```python
from build123d import *

# Parameters (mm, degrees)
ESBO_O2_R                = 8.85
RESSALTO_EXTRUS_O1_DEPTH = 6.4
ESBO_O3_R                = 8.25
CORTE_EXTRUS_O1_DEPTH    = 5
ESBO_O4_R                = 7.75
RESSALTO_EXTRUS_O2_DEPTH = 9
FILETE1_R                = 0.2
ESBO_O5_R                = 7.8
RESSALTO_EXTRUS_O3_DEPTH = 11
ESBO_O6_R                = 7.25
RESSALTO_EXTRUS_O4_DEPTH = 10.3
ESBO_O7_W                = 21.473826642
ESBO_O7_H                = 23.10287556
CORTE_EXTRUS_O2_DEPTH    = 11
ESBO_O8_W                = 2.8
ESBO_O8_H                = 0.5
RESSALTO_EXTRUS_O5_DEPTH = 8


with BuildPart() as part:
    # Esboço2 → Ressalto-extrusão1 (new body)
    with BuildSketch(Plane(origin=(0, 0, 0), x_dir=(1, 0, 0), z_dir=(0, 1, 0))):
        Circle(ESBO_O2_R)
    extrude(amount=RESSALTO_EXTRUS_O1_DEPTH)

    # Esboço3 → Corte-extrusão1 (cut)
    with BuildSketch(Plane(origin=(0, 6.4, 0), x_dir=(1, 0, 0), z_dir=(0, 1, 0))):
        Circle(ESBO_O3_R)
    extrude(amount=-CORTE_EXTRUS_O1_DEPTH, mode=Mode.SUBTRACT)

    # Esboço4 → Ressalto-extrusão2 (add)
    with BuildSketch(Plane(origin=(0, 1.4, 0), x_dir=(1, 0, 0), z_dir=(0, 1, 0))):
        Circle(ESBO_O4_R)
    extrude(amount=RESSALTO_EXTRUS_O2_DEPTH)

    # Filete1
    filete1_edges = [part.edges().sort_by_distance(p)[0] for p in [
        (-7.75, 10.4, 0),
        (-8.85, 6.4, 0),
    ]]
    fillet(filete1_edges, radius=FILETE1_R)

    # Esboço5 → Ressalto-extrusão3 (add)
    with BuildSketch(Plane.XZ):
        Circle(ESBO_O5_R)
    extrude(amount=RESSALTO_EXTRUS_O3_DEPTH)

    # Esboço6 → Ressalto-extrusão4 (add)
    with BuildSketch(Plane.XZ.offset(11)):
        Circle(ESBO_O6_R)
    extrude(amount=RESSALTO_EXTRUS_O4_DEPTH)

    # Esboço7 → Corte-extrusão2 (cut)
    with BuildSketch(Plane.XZ.offset(11)):
        Rectangle(ESBO_O7_W, ESBO_O7_H)
        Polygon((-7.25, -7.8), (-1, -7.8), (-1, -7.25), (1, -7.25), (1, -7.8), (7.25, -7.8), (7.25, 7.8), (1, 7.8), (1, 7.25), (-1, 7.25), (-1, 7.8), (-7.25, 7.8), align=None, mode=Mode.SUBTRACT)
    extrude(amount=-CORTE_EXTRUS_O2_DEPTH, mode=Mode.SUBTRACT)

    # Esboço8 → Ressalto-extrusão5 (add)
    with BuildSketch(Plane.XZ.offset(21.3)):
        with Locations((-5, 2.75)):
            Rectangle(ESBO_O8_W, ESBO_O8_H)
        with Locations((0, 2.75)):
            Rectangle(ESBO_O8_W, ESBO_O8_H)
        with Locations((5, 2.75)):
            Rectangle(ESBO_O8_W, ESBO_O8_H)
        with Locations((0, 6.25)):
            Rectangle(ESBO_O8_W, ESBO_O8_H)
        with Locations((0, -6.25)):
            Rectangle(ESBO_O8_W, ESBO_O8_H)
        with Locations((5, -2.75)):
            Rectangle(ESBO_O8_W, ESBO_O8_H)
        with Locations((0, -2.75)):
            Rectangle(ESBO_O8_W, ESBO_O8_H)
        with Locations((-5, -2.75)):
            Rectangle(ESBO_O8_W, ESBO_O8_H)
    extrude(amount=RESSALTO_EXTRUS_O5_DEPTH)


solid = part.part
```
The model under review builds one solid part; all positions refer to its coordinate system, in mm. A direction names the side the tool comes from. Round coordinates to 2 decimals unless told otherwise and drop trailing zeros. Order: outer loops, then holes, each group sorted by start corner. A loop starts at its lowest first (then second) coordinate and runs counter-clockwise, first axis right, second up.
Item 1: To check wall thickness, follow probe 1 along X at (y, z) = (4.5, 0); probe 2 along X at (y, z) = (3, 4.25). State the ranges of each line that lie inside material, in increasing order.
Working result:
probe 1: x = -8.85 to -8.25, -7.75 to 7.75, 8.25 to 8.85
probe 2: x = -7.76 to -7.07, -6.48 to 6.48, 7.07 to 7.76
Item 2: Add section C-C, the plane y = -18.5. State the section outline as (x, z) points, and give its area (3 significant figures).
Working result:
outline: circle Ø14.5 at (0, 0)
area: 165 mm2
Item 3: Add section B-B, the plane y = -8.5. State the section outline as (x, z) points, and give its area (3 significant figures).
Working result:
outline: (-7.25, -2.88) arc R7.8 ccw to (-1, -7.74) - (-1, -7.25) - (1, -7.25) - (1, -7.74) arc R7.8 ccw to (7.25, -2.88) - (7.25, 2.88) arc R7.8 ccw to (1, 7.74) - (1, 7.25) - (-1, 7.25) - (-1, 7.74) arc R7.8 ccw to (-7.25, 2.88) - close
area: 185 mm2
Item 4: Machinability: for faces 1 (the flat face through (0, -25, -6.5)), 2 (the flat face through (0, -25, 2.5)), 3 (the cylindrical face through (7.62, 3.94, 3.16)), 4 (the flat face through (0, -6, -7.25)), 5 (the flat face through (5, -25, 3)), which of the approach directions +Z, -Z, +X, -X, +Y, -Y give a long, thin tool a straight path to every point of the face, cutting with its end or side? Answer none if there is none.
Working result:
face 1: -Z, +X, -X, -Y
face 2: +X, -X, -Y
face 3: +Y
face 4: -Z, -Y
face 5: +Z, +X, -X, -Y
Item 5: For pin 1 (0.6 mm diameter, centred on y = -24, z = 3, fed in from +X); pin 2 (3 mm diameter, centred on x = 0, y = -26.5, fed in from -Z); pin 3 (5 mm diameter, centred on y = -18.5, z = 7, fed in from +X); pin 4 (8 mm diameter, centred on x = -1.5, z = 0.5, fed in from -Y), all flat-tipped, find the tip position at first contact; note any pin that passes through.
Working result:
pin 1: stops at x = 6.4
pin 2: stops at z = -6.5
pin 3: stops at x = 5.68
pin 4: stops at y = -29.3
Item 6: Draft analysis for pull direction Z (two halves, no side actions). For faces 6 (the flat face through (-5, -11, 5.6)), 7 (the flat face through (-5, -25, 3)), 8 (the flat face through (0, -25, -3)), state which applies: released by +Z, released by -Z, zero draft, split by the parting line, or undercut.
Working result:
face 6: zero draft
face 7: released by +Z
face 8: undercut
Item 7: Add section A-A, the plane y = -25. Count the separate pieces of the cut face and the enclosed holes in it, and give its area (3 significant figures).
Working result:
separate pieces: 8
enclosed holes: 0
area: 11.2 mm2
